```python
from build123d import *

# Parameters (mm, degrees)
F0_W          = 50.8
F0_H          = 50.8
F1_DEPTH      = 114.3
F2_R          = 12.7
F3_DEPTH      = 76.2
F2_R_2        = 19.05
F4_DEPTH      = 12.7
F4_DEPTH_BACK = 63.5
F5_R          = 10.16
F6_DEPTH      = 101.6
F5_W          = 50.8
F5_H          = 50.8
F7_DEPTH      = 25.4


with BuildPart() as f1:
    # F0 (on Top) → F1 (new body)
    with BuildSketch(Plane.XY):
        with Locations((-24.373119, -0.228241)):
            Rectangle(F0_W, F0_H)
    extrude(amount=F1_DEPTH)

    # F2 (on face) → F3 (cut)
    with BuildSketch(Plane.XZ.offset(25.628241)):
        with Locations((-24.373119, 57.15)):
            Circle(F2_R)
    extrude(amount=-F3_DEPTH, mode=Mode.SUBTRACT)

    # F2 (on face) → F4 (join, two sides)
    with BuildSketch(Plane.XZ.offset(25.628241)) as f4_sk:
        with Locations((-24.373119, 57.15)):
            Circle(F2_R_2)
        with Locations((-24.373119, 57.15)):
            Circle(F2_R, mode=Mode.SUBTRACT)
    extrude(amount=F4_DEPTH)
    extrude(f4_sk.sketch, amount=-F4_DEPTH_BACK)

    # F5 (on face) → F6 (join)
    with BuildSketch(Plane(origin=(-49.773119, 0, 0), x_dir=(0, -1, 0), z_dir=(-1, 0, 0))):
        with Locations((0.228241, 57.132342)):
            Circle(F5_R)
    extrude(amount=F6_DEPTH)

    # F5 (on face) → F7 (join)
    with BuildSketch(Plane(origin=(-49.773119, 0, 0), x_dir=(0, -1, 0), z_dir=(-1, 0, 0))):
        with Locations((0.228241, 57.132342)):
            Rectangle(F5_W, F5_H)
        with Locations((0.228241, 57.132342)):
            Circle(F5_R, mode=Mode.SUBTRACT)
    extrude(amount=F7_DEPTH)


solid = f1.part
```
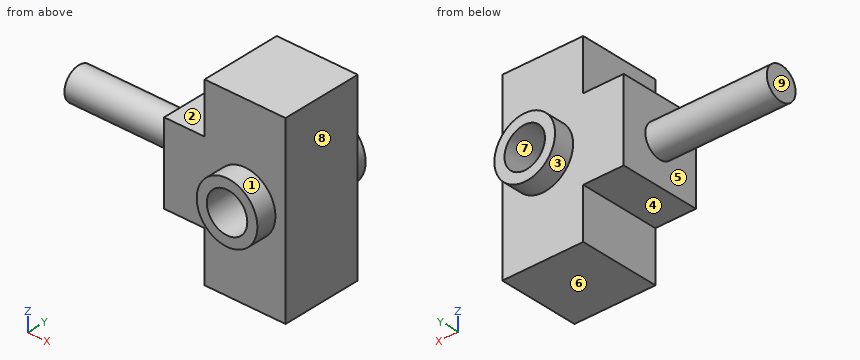
Geometry: final body of the model. Coordinates: model frame, mm. Face numbers are marked on the shaded views. A direction names the side the tool comes from. Round coordinates to 2 decimals unless told otherwise and drop trailing zeros. Order: outer loops, then holes, each group sorted by start corner. A loop starts at its lowest first (then second) coordinate and runs counter-clockwise, first axis right, second up. Notation, with made-up numbers: (7.5, 49.25) -> (22.5, 49.25) arc R16 ccw to (22.5, 56.25) -> close; hole circle Ø11 at (10.5, -18). An arc over 180 degrees is marked (long way). Use CSV: the item, a comma, the result in double quotes. Start each with the question number.
1) Section D-D (x = -39.5). Return the cut outline in (y, z).
2) Material intervals for line 1 along Z through (x, y) = (-23.5, 21); line 2 along X through (y, z) = (13, 57); line 3 along X through (y, z) = (-10, 80), sorted ascending. Write a range as from..to.
3) First-contact query: pin 1 Ø2 at (y, z) = (-23, 34.5) entering from -X; pin 2 Ø3 at (x, z) = (-49, 49.5) entering from -Y; pin 3 Ø1.5 at (x, y) = (-92, 0) entering from -Z; pin 4 Ø4 at (x, z) = (-67, 28.5) entering from -Y. Flat tips, straight axial feed; report the tip coordinate or a pass-through.
4) Section B-B (z = 54). Return the cut outline in (x, y).
5) Set-up query: the marked faces 1, 2, 3, 4 and 5. Return all of +Z, -Z, +X, -X, +Y, -Y with unobstructed straight access to the full face (end or side cutting, diameter ignored); none if empty.
6) Section A-A (y = -13). Return the cut outline in (x, z).
7) Section C-C (z = 90.5). Return the cut outline in (x, y).
8) Draft query along X for the marked faces 6, 7, 8 and 9. Return one class per face: +X half, -X half, draft (parallel to the pull), parting line (faces both ways), or undercut.
Returned:
1,outline,"(-38.33, 45.57) -> (-25.63, 45.57) -> (-25.63, 0) -> (25.17, 0) -> (25.17, 45.57) -> (37.87, 45.57) -> (37.87, 68.73) -> (25.17, 68.73) -> (25.17, 114.3) -> (-25.63, 114.3) -> (-25.63, 68.73) -> (-38.33, 68.73) -> close"
2,line 1,"z = 0..44.48, 69.82..114.3"
2,line 2,"x = -75.17..-37.07, -11.67..1.03"
2,line 3,"x = -75.17..1.03"
3,pin 1,"stops at x = -75.17"
3,pin 2,"stops at y = -25.63"
3,pin 3,"stops at z = 46.97"
3,pin 4,"passes through"
4,outline,"(-151.37, -9.89) -> (-75.17, -9.89) -> (-75.17, -25.63) -> (-43.16, -25.63) -> (-43.16, -38.33) -> (-36.68, -38.33) -> (-36.68, 37.87) -> (-43.16, 37.87) -> (-43.16, 25.17) -> (-75.17, 25.17) -> (-75.17, 9.44) -> (-151.37, 9.44) -> close; (-12.07, -38.33) -> (-5.59, -38.33) -> (-5.59, -25.63) -> (1.03, -25.63) -> (1.03, 25.17) -> (-5.59, 25.17) -> (-5.59, 37.87) -> (-12.07, 37.87) -> close"
5,face 1,"-Y"
5,face 2,"+Z, -X, +Y, -Y"
5,face 3,"+Y"
5,face 4,"-Z, -X, +Y, -Y"
5,face 5,"-X"
6,outline,"(-75.17, 31.73) -> (-49.77, 31.73) -> (-49.77, 0) -> (1.03, 0) -> (1.03, 114.3) -> (-49.77, 114.3) -> (-49.77, 82.53) -> (-75.17, 82.53) -> close; hole circle Ø25.4 at (-24.37, 57.15)"
7,outline,"(-49.77, -25.63) -> (1.03, -25.63) -> (1.03, 25.17) -> (-49.77, 25.17) -> close"
8,face 6,"draft"
8,face 7,"undercut"
8,face 8,"+X half"
8,face 9,"-X half"
